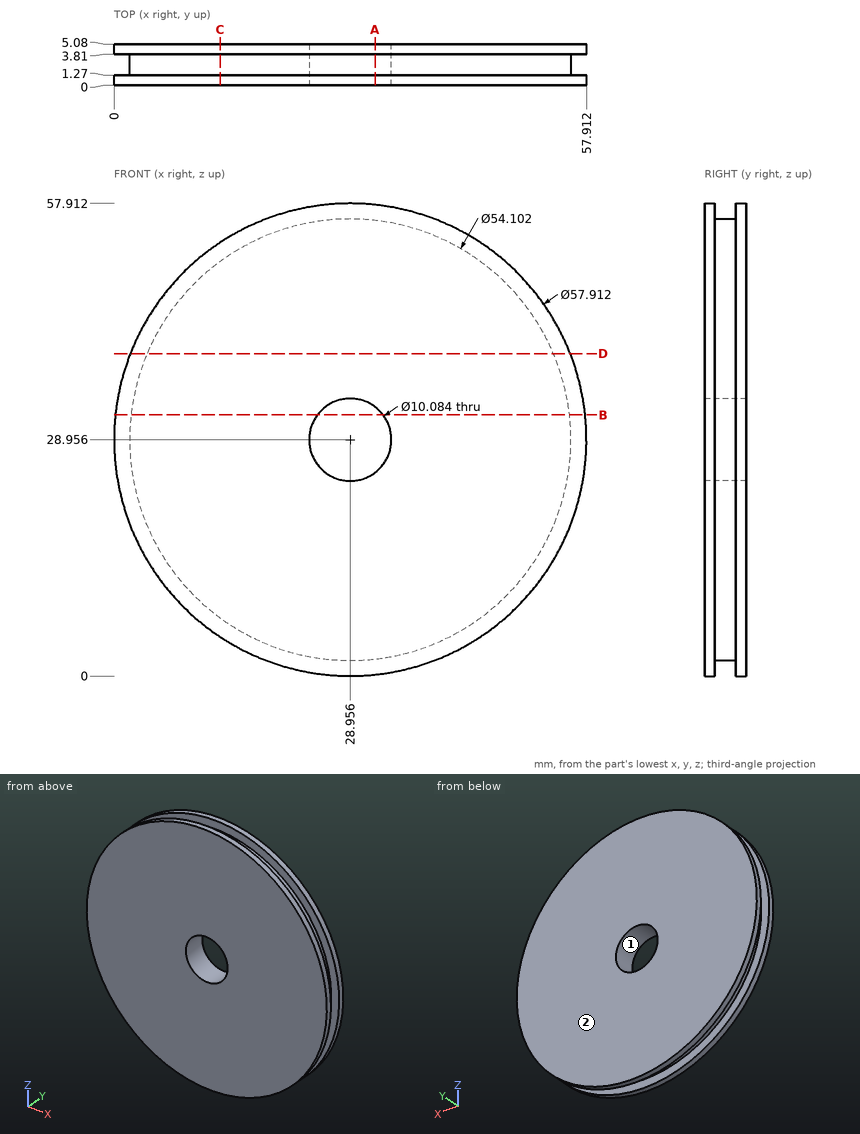
Can you work these out from the drawing? Everything is in mm from the part's minimum corner. Give positions to 0.01 mm unless a question says otherwise; leave off trailing zeros. Loops run counter-clockwise (first coordinate to the right, second up) from the corner with the lowest first, then second, coordinate; pieces in that order, holes last. Notation, with made-up numbers: (-15, 27) -> (40, 27) arc R6 ccw to (40, 35) -> close; hole circle Ø4 at (-38.5, 57). An arc over 180 degrees is marked (long way). Return JSON: item names as keys, results as strings.
Item 1: If we section it at C-C on x = 13: List the corners of the cut face in (y, z) for me, plus the area to 3 significant figures.
Geometry results:
{"outline": "(0, 4.79) -> (1.27, 4.79) -> (1.27, 7.11) -> (3.81, 7.11) -> (3.81, 4.79) -> (5.08, 4.79) -> (5.08, 53.12) -> (3.81, 53.12) -> (3.81, 50.8) -> (1.27, 50.8) -> (1.27, 53.12) -> (0, 53.12) -> close", "area": "234 mm²"}
Item 2: If we section it at B-B on z = 32: List the corners of the cut face in (x, y) for me (1 decimal), plus the area to 3 significant figures.
Geometry results:
{"outline": "(0.2, 0) -> (24.9, 0) -> (24.9, 5.1) -> (0.2, 5.1) -> (0.2, 3.8) -> (2.1, 3.8) -> (2.1, 1.3) -> (0.2, 1.3) -> close; (33, 0) -> (57.8, 0) -> (57.8, 1.3) -> (55.8, 1.3) -> (55.8, 3.8) -> (57.8, 3.8) -> (57.8, 5.1) -> (33, 5.1) -> close", "area": "242 mm²"}
Item 3: If we section it at D-D on z = 39.5: List the corners of the cut face in (x, y) for me.
Geometry results:
{"outline": "(1.99, 0) -> (55.92, 0) -> (55.92, 1.27) -> (53.87, 1.27) -> (53.87, 3.81) -> (55.92, 3.81) -> (55.92, 5.08) -> (1.99, 5.08) -> (1.99, 3.81) -> (4.04, 3.81) -> (4.04, 1.27) -> (1.99, 1.27) -> close"}
Item 4: We'd pull the mould along Z, two halves only. Please class the marked faces 1 and 2: +Z half, -Z half, draft (parallel to the pull), parting line (faces both ways), or undercut.
Geometry results:
{"face 1": "undercut", "face 2": "draft"}
Item 5: If we section it at A-A on x = 32: List the corners of the cut face in (y, z) for me (1 decimal).
Geometry results:
{"outline": "(0, 0.2) -> (1.3, 0.2) -> (1.3, 2.1) -> (3.8, 2.1) -> (3.8, 0.2) -> (5.1, 0.2) -> (5.1, 24.9) -> (0, 24.9) -> close; (0, 33) -> (5.1, 33) -> (5.1, 57.8) -> (3.8, 57.8) -> (3.8, 55.8) -> (1.3, 55.8) -> (1.3, 57.8) -> (0, 57.8) -> close"}
Item 6: I need wall thicknesses on L1, parallel to Y at x = 18, z = 3.5; L2, parallel to Z at x = 33, y = 2.55 (1 decimal); L3, parallel to X at y = 1.35, z = 26.5 (1 decimal). Which ranges of each line are inside material? Lowest first, please. Write a range as from..to.
Geometry results:
{"L1": "y = 0..1.27, 3.81..5.08", "L2": "z = 2.2..25.9, 32..55.7", "L3": "x = 2..24.6, 33.4..55.9"}
Item 7: I'm going to push flat-ended pins straight in: pin 1 (3 mm diameter, centred on y = 2.5, z = 11.5, fed in from +X); pin 2 (6 mm diameter, centred on x = 28.956, z = 28.956, fed in from -Y); pin 3 (2 mm diameter, centred on x = 33.5, y = 0.5, fed in from -Z). Where does each tip first touch, or does it pass through?
Geometry results:
{"pin 1": "stops at x = 52.68", "pin 2": "passes through", "pin 3": "stops at z = 0.22"}
